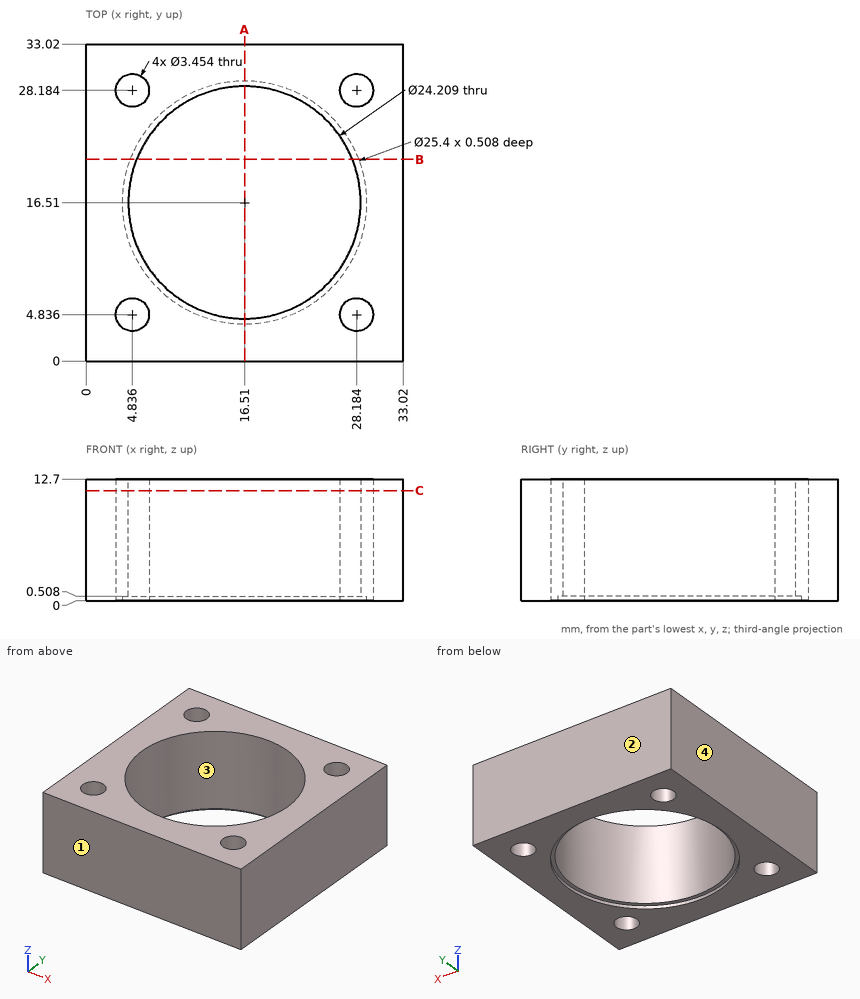
The figure shows three views and two pictorial views of one solid part (mm, origin at its lowest corner). Answer the questions. Round coordinates to 2 decimals unless told otherwise and drop trailing zeros. Loops run counter-clockwise (first coordinate to the right, second up) from the corner with the lowest first, then second, coordinate; pieces in that order, holes last. Notation, with made-up numbers: M 37.5,-38.75 L 41.5,-38.75 A18 cw 41.5,-30.75 Z; hole C 10,88.5 d11. An arc over 180 degrees is marked long. Use CSV: the item, a comma, the result in double quotes.
Q1. Section A-A, the plane x = 16.51 is taken. Determine the outline of the cut face in (y, z) (1 decimal).
Determined:
outline,"M 0,0 L 3.8,0 L 3.8,0.5 L 4.4,0.5 L 4.4,12.7 L 0,12.7 Z; M 28.6,0.5 L 29.2,0.5 L 29.2,0 L 33,0 L 33,12.7 L 28.6,12.7 Z"
Q2. Consider L1, parallel to Y at x = 16.51, z = 4 (1 decimal); L2, parallel to Y at x = 29, z = 5; L3, parallel to Y at x = 16.51, z = 0.3. Determine where each line is inside the solid, lowest interval first.
Determined:
L1,"0 to 4.4, 28.6 to 33"
L2,"0 to 3.31, 6.36 to 26.66, 29.71 to 33.02"
L3,"0 to 3.81, 29.21 to 33.02"
Q3. The mould has two halves that part along Y. Classify the marked faces 1, 2, 3 and 4: pulls with the +Y half, pulls with the -Y half, needs draft (parallel to the pull), parting line crosses it, or undercut.
Determined:
face 1,"pulls with the -Y half"
face 2,"pulls with the +Y half"
face 3,"undercut"
face 4,"needs draft"
Q4. Section B-B, the plane y = 21 is taken. Determine the outline of the cut face in (x, z).
Determined:
outline,"M 0,0 L 4.63,0 L 4.63,0.51 L 5.27,0.51 L 5.27,12.7 L 0,12.7 Z; M 27.75,0.51 L 28.39,0.51 L 28.39,0 L 33.02,0 L 33.02,12.7 L 27.75,12.7 Z"
Q5. Section C-C, the plane z = 11.5 is taken. Determine the outline of the cut face in (x, y) (1 decimal).
Determined:
outline,"M 0,0 L 33,0 L 33,33 L 0,33 Z; hole C 4.8,4.8 d3.5; hole C 4.8,28.2 d3.5; hole C 16.5,16.5 d24.2; hole C 28.2,4.8 d3.5; hole C 28.2,28.2 d3.5"
Q6. This flat-tipped pin is pushed along its axis until it touches: pin 1 (2 mm diameter, centred on x = 27, y = 19.5, fed in from -Z). Where does it stop, or does it pass through?
Determined:
pin 1,"through"
